Could you check a few things on this model? Use its own coordinates, in mm. Give positions to 0.01 mm unless a question says otherwise; leave off trailing zeros. Write each loop counter-clockwise with the first axis right and the second up, starting at its lowest first coordinate (ties: lowest second). Pieces come first, ordered by that corner, then holes. Notation, with made-up numbers: (15, 17) - (36, 17) arc R17 cw to (36, 34) - close; hole circle Ø4 at (50, -32.5). An arc over 180 degrees is marked (long way). Answer in a Markdown table with one row per item.
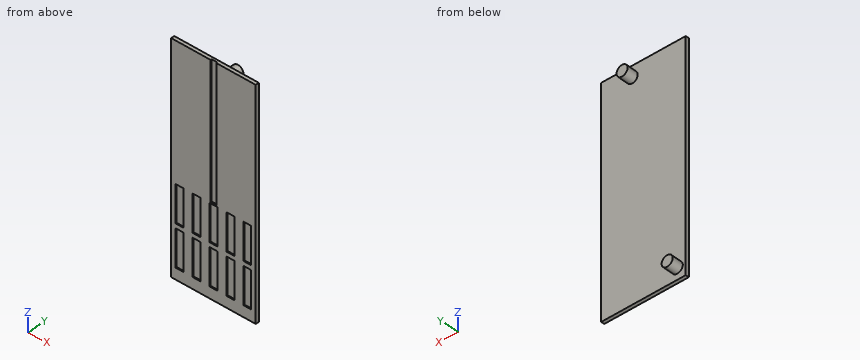
from build123d import *

# Parameters (mm, degrees)
SKETCH1_W           = 75
SKETCH1_H           = 3
BOSS_EXTRUDE1_DEPTH = 200
SKETCH2_R           = 4.9
BOSS_EXTRUDE2_DEPTH = 10
SKETCH3_W           = 5
SKETCH3_H           = 119
CUT_EXTRUDE1_DEPTH  = 1
SKETCH4_W           = 7
SKETCH4_H           = 33
CUT_EXTRUDE2_DEPTH  = 1


with BuildPart() as part:
    # Sketch1 → Boss-Extrude1 (new body)
    with BuildSketch(Plane.XY):
        with Locations((37.5, 1.5)):
            Rectangle(SKETCH1_W, SKETCH1_H)
    extrude(amount=BOSS_EXTRUDE1_DEPTH)

    # Sketch2 → Boss-Extrude2 (add)
    with BuildSketch(Plane(origin=(0, 3, 0), x_dir=(1, 0, 0), z_dir=(0, 1, 0))):
        with Locations(Location((7.5, -10, 0), (0, 0, 90))):
            Circle(SKETCH2_R)
        with Locations(Location((47.5, -190, 0), (0, 0, 90))):
            Circle(SKETCH2_R)
    extrude(amount=BOSS_EXTRUDE2_DEPTH)

    # Sketch3 → Cut-Extrude1 (cut)
    with BuildSketch(Plane.XZ):
        with Locations((37.5, 140.5)):
            Rectangle(SKETCH3_W, SKETCH3_H)
    extrude(amount=-CUT_EXTRUDE1_DEPTH, mode=Mode.SUBTRACT)

    # Sketch4 → Cut-Extrude2 (cut)
    with BuildSketch(Plane.XZ):
        with Locations((7.5, 26.5)):
            Rectangle(SKETCH4_W, SKETCH4_H)
        with Locations((7.5, 63.5)):
            Rectangle(SKETCH4_W, SKETCH4_H)
        with Locations((22.5, 26.5)):
            Rectangle(SKETCH4_W, SKETCH4_H)
        with Locations((22.5, 63.5)):
            Rectangle(SKETCH4_W, SKETCH4_H)
        with Locations((37.5, 26.5)):
            Rectangle(SKETCH4_W, SKETCH4_H)
        with Locations((37.5, 63.5)):
            Rectangle(SKETCH4_W, SKETCH4_H)
        with Locations((52.5, 26.5)):
            Rectangle(SKETCH4_W, SKETCH4_H)
        with Locations((52.5, 63.5)):
            Rectangle(SKETCH4_W, SKETCH4_H)
        with Locations((67.5, 26.5)):
            Rectangle(SKETCH4_W, SKETCH4_H)
        with Locations((67.5, 63.5)):
            Rectangle(SKETCH4_W, SKETCH4_H)
    extrude(amount=-CUT_EXTRUDE2_DEPTH, mode=Mode.SUBTRACT)


solid = part.part
1) If I drill on line 1 (Y direction, x = 22.5, z = 46.5); line 2 (X direction, y = 0.5, z = 146); line 3 (Y direction, x = 25.5, z = 62.5), over which ranges is the centre line in solid material (lowest first)?
Check values:
| item | result |
|---|---|
| line 1 | y = 0 to 3 |
| line 2 | x = 0 to 35, 40 to 75 |
| line 3 | y = 1 to 3 |
2) Will these pins go through, and if not, where does the flat tip stop? P1, Ø3, axis at x = 45, z = 37, coming from the +Y side; P2, Ø3.5, axis at x = 37, z = 20, coming from the -Y side.
Check values:
| item | result |
|---|---|
| P1 | stops at y = 3 |
| P2 | stops at y = 1 |
3) Imagine slicing it at B-B (y = 7.5). List the corners of the cut face in (x, z) for me, then the cut area to 3 significant figures.
Check values:
| item | result |
|---|---|
| outline | circle Ø9.8 at (7.5, 10); circle Ø9.8 at (47.5, 190) |
| area | 151 mm2 |
4) Imagine slicing it at C-C (z = 170). List the corners of the cut face in (x, y) for me, then the cut area to 3 significant figures.
Check values:
| item | result |
|---|---|
| outline | (0, 0) - (35, 0) - (35, 1) - (40, 1) - (40, 0) - (75, 0) - (75, 3) - (0, 3) - close |
| area | 220 mm2 |
5) Imagine slicing it at A-A (x = 7.5). List the corners of the cut face in (y, z) for me.
Check values:
| item | result |
|---|---|
| outline | (0, 0) - (3, 0) - (3, 5.1) - (13, 5.1) - (13, 14.9) - (3, 14.9) - (3, 200) - (0, 200) - (0, 80) - (1, 80) - (1, 47) - (0, 47) - (0, 43) - (1, 43) - (1, 10) - (0, 10) - close |
6) Imagine slicing it at D-D (z = 73). List the corners of the cut face in (x, y) for me, then the cut area to 3 significant figures.
Check values:
| item | result |
|---|---|
| outline | (0, 0) - (4, 0) - (4, 1) - (11, 1) - (11, 0) - (19, 0) - (19, 1) - (26, 1) - (26, 0) - (34, 0) - (34, 1) - (41, 1) - (41, 0) - (49, 0) - (49, 1) - (56, 1) - (56, 0) - (64, 0) - (64, 1) - (71, 1) - (71, 0) - (75, 0) - (75, 3) - (0, 3) - close |
| area | 190 mm2 |
